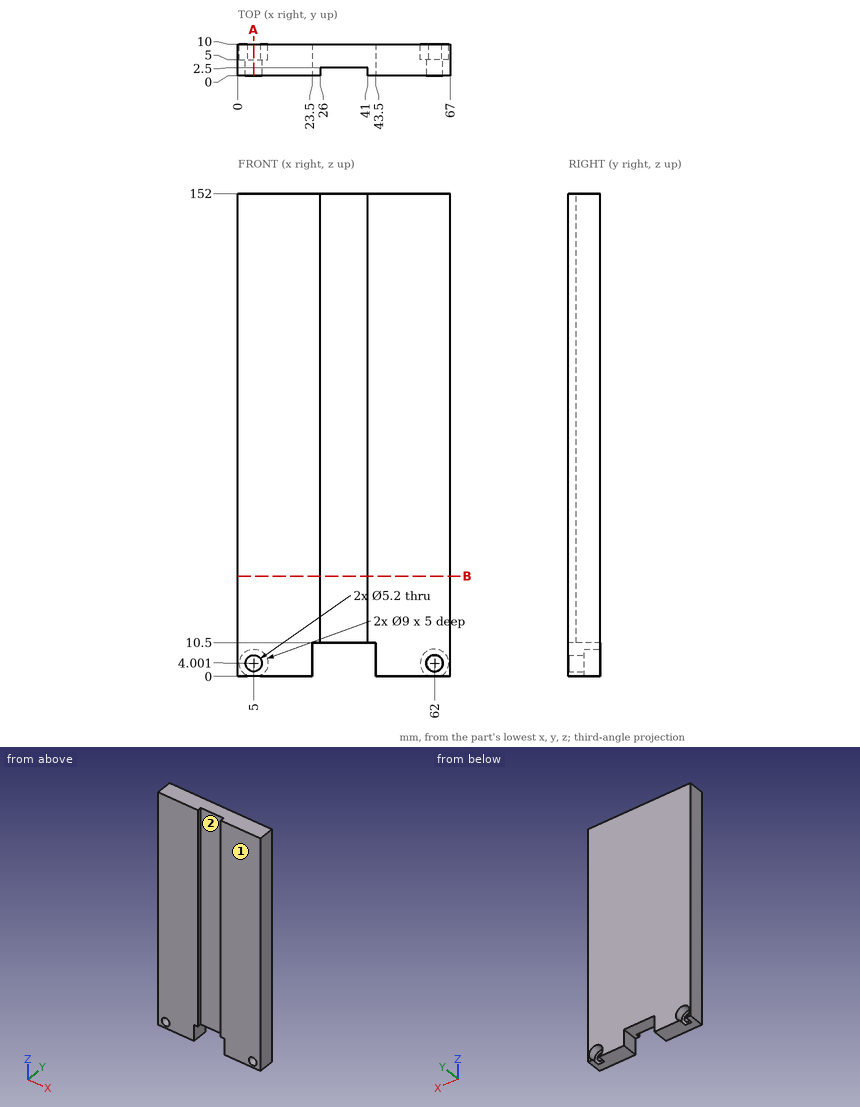
For this review, use the dimensioned drawing (mm, ordinates from the lowest corner) and the shaded views. Give positions to 0.01 mm unless a question says otherwise; leave off trailing zeros. Order: outer loops, then holes, each group sorted by start corner. A loop starts at its lowest first (then second) coordinate and runs counter-clockwise, first axis right, second up. Notation, with made-up numbers: (-8.5, 78) - (42.5, 78) arc R18 cw to (42.5, 107) - close; hole circle Ø1 at (71.5, 74). An arc over 180 degrees is marked (long way). Use a Markdown table: item, result. Add a question column.
(1) Add section B-B on z = 31.5. Give the boundary of the cut face in (x, y).
(2) Add section A-A on x = 5. Give the boundary of the cut face in (y, z).
(3) Clearance check with flat-ended pins moving along their axes: P1, Ø5.5, axis at x = 5, z = 4, coming from the -Y side; P2, Ø3, axis at x = 40, y = 4.5, coming from the -Z side; P3, Ø2.5, axis at x = 5.5, z = 2.5, coming from the +Y side. State where each tip first meets the part, or that it passes through.
(4) Mouldability with a two-part tool opening along X and no side actions: class the marked faces 1 and 2 as +X half, -X half, draft (parallel to the pull), parting line (faces both ways), or undercut.
(5) Wall thickness on probe 1 along X at (y, z) = (1.75, 45); probe 2 along Z at (x, y) = (62, 1.95); probe 3 along Y at (x, z) = (33.5, 131): over which ranges is each line inside the solid? List them lowest first. Write a range as [from, to].
Report:
| question | item | result |
|---|---|---|
| 1 | outline | (0, 0) - (26, 0) - (26, 2.5) - (41, 2.5) - (41, 0) - (67, 0) - (67, 10) - (0, 10) - close |
| 2 | outline | (0, 0) - (5, 0) - (5, 1.4) - (0, 1.4) - close; (0, 6.6) - (5, 6.6) - (5, 8.5) - (10, 8.5) - (10, 152) - (0, 152) - close |
| 3 | P1 | stops at y = 0 |
| 3 | P2 | stops at z = 10.5 |
| 3 | P3 | stops at y = 5 |
| 4 | face 1 | draft |
| 4 | face 2 | undercut |
| 5 | probe 1 | x = [0, 26], [41, 67] |
| 5 | probe 2 | z = [0, 1.4], [6.6, 152] |
| 5 | probe 3 | y = [2.5, 10] |
